from build123d import *

# Parameters (mm, degrees)
SKETCH1_W                = 20
SKETCH1_H                = 70
BOSS_EXTRUDE1_DEPTH      = 10
SKETCH2_W                = 20.25
SKETCH2_H                = 5.1
CUT_EXTRUDE1_DEPTH       = 1
CUT_EXTRUDE1_DEPTH_BACK  = 21
SKETCH3_R                = 4.15
CUT_EXTRUDE2_DEPTH       = 11
BOSS_EXTRUDE2_DEPTH      = 7.5
BOSS_EXTRUDE2_DEPTH_BACK = 27.5
CHAMFER1_SIZE            = 1
CHAMFER1_SIZE2           = 0.577350269
CHAMFER1_PART_2_SIZE     = 1
CHAMFER1_PART_2_SIZE2    = 0.577350269


with BuildPart() as part:
    # Sketch1 → Boss-Extrude1 (new body)
    with BuildSketch(Plane(origin=(0, 0, 0), x_dir=(1, 0, 0), z_dir=(0, 1, 0))):
        Rectangle(SKETCH1_W, SKETCH1_H)
    extrude(amount=BOSS_EXTRUDE1_DEPTH)

    # Sketch2 → Cut-Extrude1 (cut, two sides)
    with BuildSketch(Plane(origin=(10, 0, 0), x_dir=(0, 0, -1), z_dir=(1, 0, 0))) as cut_extrude1_sk:
        with Locations((0, 2.55)):
            Rectangle(SKETCH2_W, SKETCH2_H)
    extrude(amount=CUT_EXTRUDE1_DEPTH, mode=Mode.SUBTRACT)
    extrude(cut_extrude1_sk.sketch, amount=-CUT_EXTRUDE1_DEPTH_BACK, mode=Mode.SUBTRACT)

    # Sketch3 → Cut-Extrude2 (cut, through all)
    with BuildSketch(Plane.XZ):
        with Locations(Location((0, 25, 0), (0, 0, 270))):  # turned: the seam where the file's is
            Circle(SKETCH3_R)
        with Locations(Location((0, -25, 0), (0, 0, 270))):  # turned: the seam where the file's is
            Circle(SKETCH3_R)
    extrude(amount=-CUT_EXTRUDE2_DEPTH, mode=Mode.SUBTRACT)

    # Sketch4 → Boss-Extrude2 (add, two sides)
    with BuildSketch(Plane(origin=(10, 0, 0), x_dir=(0, 0, -1), z_dir=(1, 0, 0))) as boss_extrude2_sk:
        Polygon((-10.125, 0), (-15.005, 0), (-15.005, 10), (15.005, 10), (15.005, 0), (10.125, 0), (10.125, 5.1), (-10.125, 5.1), align=None)
    extrude(amount=BOSS_EXTRUDE2_DEPTH)
    extrude(boss_extrude2_sk.sketch, amount=-BOSS_EXTRUDE2_DEPTH_BACK)

    # Chamfer1
    chamfer1_edges = [part.edges().sort_by_distance(p)[0] for p in [
        (0, 10, 29.15),
    ]]
    chamfer1_side = [part.faces().sort_by_distance(p)[0] for p in [
        (0, 5, 29.15),
    ]]
    chamfer(chamfer1_edges, length=CHAMFER1_SIZE, length2=CHAMFER1_SIZE2, reference=chamfer1_side[0])

    # Chamfer1 part 2
    chamfer1_part_2_edges = [part.edges().sort_by_distance(p)[0] for p in [
        (0, 10, -20.85),
    ]]
    chamfer1_part_2_side = [part.faces().sort_by_distance(p)[0] for p in [
        (0, 5, -20.85),
    ]]
    chamfer(chamfer1_part_2_edges, length=CHAMFER1_PART_2_SIZE, length2=CHAMFER1_PART_2_SIZE2, reference=chamfer1_part_2_side[0])


solid = part.part
Read the model definition and answer for the solid it produces. Units are mm, in the model's axes. A direction names the side the tool comes from. Round coordinates to 2 decimals unless told otherwise and drop trailing zeros. Write each loop counter-clockwise with the first axis right and the second up, starting at its lowest first coordinate (ties: lowest second). Pieces come first, ordered by that corner, then holes. Notation, with made-up numbers: M -7.5,44 L 31.5,44 A14 cw 31.5,70 Z; hole C -23.5,88 d9. An arc over 180 degrees is marked long. Use a Markdown table: item, result.
1) Straight lines are drawn through the part: line 1 along X through (y, z) = (3.5, -25); line 2 along Z through (x, y) = (-14, 4) (3 decimals); line 3 along Z through (x, y) = (-12, 5.5) (3 decimals). For each, find the intervals that lie inside material, in ascending order. Write a range as [from, to].
Answers follow:
| item | result |
|---|---|
| line 1 | x = [-10, -4.15], [4.15, 10] |
| line 2 | z = [-15.005, -10.125], [10.125, 15.005] |
| line 3 | z = [-15.005, 15.005] |
2) The part is cut by section C-C (x = 0). Write down the section's boundary in (y, z) (3 decimals), plus the area to 3 significant figures.
Answers follow:
| item | result |
|---|---|
| outline | M 0,-35 L 10,-35 L 10,-29.727 L 9,-29.15 L 0,-29.15 Z; M 0,-20.85 L 9,-20.85 L 10,-20.273 L 10,20.273 L 9,20.85 L 0,20.85 L 0,10.125 L 5.1,10.125 L 5.1,-10.125 L 0,-10.125 Z; M 0,29.15 L 9,29.15 L 10,29.727 L 10,35 L 0,35 Z |
| area | 430 mm2 |
3) A tool of negligible diameter and unlimited length cuts with its end or side. For faces 1 (the flat face through (-14, 5, 15.005)), 2 (the flat face through (0, 3, 10.125)), 3 (the flat face through (-10, 5, -25)), from which of +Z, -Z, +X, -X, +Y, -Y can it reach the whole face along a straight path? Write none if from no direction.
Answers follow:
| item | result |
|---|---|
| face 1 | +Z, -X, +Y, -Y |
| face 2 | +X, -X, -Y |
| face 3 | -Z, -X, +Y, -Y |
4) Flat-ended cylindrical pins translate along their axes: pin 1 (6 mm diameter, centred on x = -15, y = 3.5, fed in from -Z) (3 decimals); pin 2 (3 mm diameter, centred on y = 3, z = -21, fed in from +X); pin 3 (3 mm diameter, centred on y = 7, z = 24.5, fed in from -X). Find the tip coordinate at first contact, or state that the pin passes through.
Answers follow:
| item | result |
|---|---|
| pin 1 | stops at z = -15.005 |
| pin 2 | stops at x = 10 |
| pin 3 | stops at x = -10 |
5) The part is cut by section D-D (y = 6.75). Write down the section's boundary in (x, z) (3 decimals).
Answers follow:
| item | result |
|---|---|
| outline | M -17.5,-15.005 L -10,-15.005 L -10,-35 L 10,-35 L 10,-15.005 L 17.5,-15.005 L 17.5,15.005 L 10,15.005 L 10,35 L -10,35 L -10,15.005 L -17.5,15.005 Z; hole C 0,-25 d8.3; hole C 0,25 d8.3 |
6) The part is cut by section A-A (y = 2.25). Write down the section's boundary in (x, z) (3 decimals).
Answers follow:
| item | result |
|---|---|
| outline | M -17.5,-15.005 L -10,-15.005 L -10,-35 L 10,-35 L 10,-15.005 L 17.5,-15.005 L 17.5,-10.125 L -17.5,-10.125 Z; M -17.5,10.125 L 17.5,10.125 L 17.5,15.005 L 10,15.005 L 10,35 L -10,35 L -10,15.005 L -17.5,15.005 Z; hole C 0,-25 d8.3; hole C 0,25 d8.3 |
7) For a pull along Z with two mould halves and no side action, classify faces 4 (the flat face through (0, 3, -10.125)), 5 (the flat face through (17.5, 6, 0)), 6 (the flat face through (0, 5, 35)) as pulls with the +Z half, pulls with the -Z half, needs draft (parallel to the pull), parting line crosses it, or undercut.
Answers follow:
| item | result |
|---|---|
| face 4 | undercut |
| face 5 | needs draft |
| face 6 | pulls with the +Z half |
8) The part is cut by section B-B (z = 25). Write down the section's boundary in (x, y), plus the area to 3 significant figures.
Answers follow:
| item | result |
|---|---|
| outline | M -10,0 L -4.15,0 L -4.15,9 L -4.73,10 L -10,10 Z; M 4.15,0 L 10,0 L 10,10 L 4.73,10 L 4.15,9 Z |
| area | 116 mm2 |
